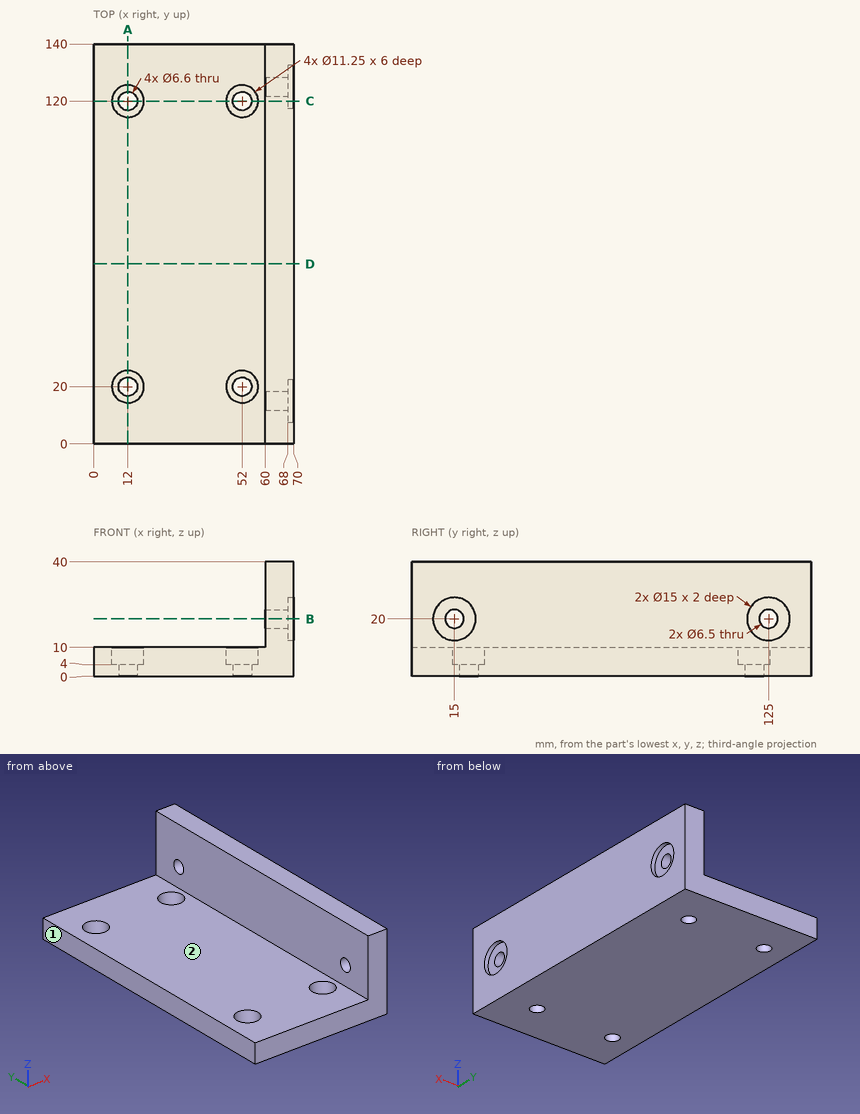
Could you check a few things on this drawing? It's one solid part, dimensions in mm from its lowest x, y, z. A direction names the side the tool comes from. Coordinates: 2 decimals unless noted, no trailing zeros. Write each loop counter-clockwise with the first axis right and the second up, starting at its lowest first coordinate (ties: lowest second). Pieces come first, ordered by that corner, then holes. Notation, with made-up numbers: (17, 76) - (45, 76) arc R29 ccw to (45, 96) - close; hole circle Ø1 at (27.5, 59). An arc over 180 degrees is marked (long way). Return JSON: item names as keys, results as strings. Group by question number.
Item 1: If we section it at D-D (y = 63): Write out the boundary of the cut face in (x, z).
Item 2: Which directions (+Z, -Z, +X, -X, +Y, -Y) give clear straight access to the entire face, cutting with the end or side of a thin tool? Please do the marked faces 1 and 2.
Item 3: If we section it at B-B (z = 20): Write out the boundary of the cut face in (x, y), then the cut area to 3 significant figures.
Item 4: I'm going to push flat-ended pins straight in: pin 1 Ø7 at (x, y) = (52, 120) entering from +Z; pin 2 Ø17 at (y, z) = (125, 20) entering from -X; pin 3 Ø5 at (x, y) = (31, 32) entering from +Z; pin 4 Ø4 at (y, z) = (15, 20) entering from +X. Where does each tip first touch, or does it pass through?
Item 5: If we section it at A-A (x = 12): Write out the boundary of the cut face in (y, z) (3 decimals), then the cut area to 3 significant figures.
Item 6: If we section it at C-C (y = 120): Write out the boundary of the cut face in (x, z) (3 decimals).
Item 7: Please list where these lines run through material, in increasing order: probe 1 along Y at (x, z) = (12, 8.2) (3 decimals); probe 2 along Y at (x, z) = (53.5, 8); probe 3 along Z at (x, y) = (66.25, 15).
Return value:
{
 "1": {"outline": "(0, 0) - (70, 0) - (70, 40) - (60, 40) - (60, 10) - (0, 10) - close"},
 "2": {"face 1": "+Z, -Z, -X, +Y, -Y", "face 2": "+Z, -X, +Y, -Y"},
 "3": {"outline": "(60, 0) - (70, 0) - (70, 7.5) - (68, 7.5) - (68, 11.75) - (60, 11.75) - close; (60, 18.25) - (68, 18.25) - (68, 22.5) - (70, 22.5) - (70, 117.5) - (68, 117.5) - (68, 121.75) - (60, 121.75) - close; (60, 128.25) - (68, 128.25) - (68, 132.5) - (70, 132.5) - (70, 140) - (60, 140) - close", "area": "1,240 mm^2"},
 "4": {"pin 1": "stops at z = 4", "pin 2": "stops at x = 60", "pin 3": "stops at z = 10", "pin 4": "passes through"},
 "5": {"outline": "(0, 0) - (16.7, 0) - (16.7, 4) - (14.375, 4) - (14.375, 10) - (0, 10) - close; (23.3, 0) - (116.7, 0) - (116.7, 4) - (114.375, 4) - (114.375, 10) - (25.625, 10) - (25.625, 4) - (23.3, 4) - close; (123.3, 0) - (140, 0) - (140, 10) - (125.625, 10) - (125.625, 4) - (123.3, 4) - close", "area": "1,210 mm^2"},
 "6": {"outline": "(0, 0) - (8.7, 0) - (8.7, 4) - (6.375, 4) - (6.375, 10) - (0, 10) - close; (15.3, 0) - (48.7, 0) - (48.7, 4) - (46.375, 4) - (46.375, 10) - (17.625, 10) - (17.625, 4) - (15.3, 4) - close; (55.3, 0) - (70, 0) - (70, 14.41) - (68, 14.41) - (68, 25.59) - (70, 25.59) - (70, 40) - (60, 40) - (60, 10) - (57.625, 10) - (57.625, 4) - (55.3, 4) - close"},
 "7": {"probe 1": "y = 0 to 14.375, 25.625 to 114.375, 125.625 to 140", "probe 2": "y = 0 to 14.58, 25.42 to 114.58, 125.42 to 140", "probe 3": "z = 0 to 16.75, 23.25 to 40"}
}
